from build123d import *

# Parameters (mm, degrees)
BOSS_EXTRUDE1_DEPTH = 40
SKETCH2_R           = 1.7
CUT_EXTRUDE1_DEPTH  = 28.75
SKETCH4_R           = 1.7
SKETCH4_R_2         = 11
CUT_EXTRUDE2_DEPTH  = 20
CHAMFER1_SIZE       = 1
CUT_EXTRUDE3_REACH  = 159.067
SKETCH5_R           = 3.3


with BuildPart() as part:
    # Sketch1 → Boss-Extrude1 (new body)
    with BuildSketch(Plane(origin=(0, 0, 0), x_dir=(1, 0, 0), z_dir=(0, 1, 0))):
        with BuildLine():
            Line((23.75, 120.769174208), (23.75, 134.895099729))
            Line((23.75, 134.895099729), (21.25, 134.895099729))
            Line((21.25, 134.895099729), (21.25, 123.995190528))
            ThreePointArc((21.25, 123.995190528), (17.839743095, 119.73175291), (18.223690728, 114.285714286))
            ThreePointArc((18.223690728, 114.285714286), (18.048629784, 111.396432549), (15.513167019, 110))
            Line((15.513167019, 110), (-15.513167019, 110))
            ThreePointArc((-15.513167019, 110), (-18.048629784, 111.396432549), (-18.223690728, 114.285714286))
            ThreePointArc((-18.223690728, 114.285714286), (-17.839743095, 119.73175291), (-21.25, 123.995190528))
            Line((-21.25, 123.995190528), (-21.25, 134.895099729))
            Line((-21.25, 134.895099729), (-23.75, 134.895099729))
            Line((-23.75, 134.895099729), (-23.75, 120.769174208))
            ThreePointArc((-23.75, 120.769174208), (-25, 114), (-26.25, 120.769174208))
            Line((-26.25, 120.769174208), (-26.25, 134.895099729))
            Line((-26.25, 134.895099729), (-28.75, 134.895099729))
            Line((-28.75, 134.895099729), (-28.75, 123.995190528))
            ThreePointArc((-28.75, 123.995190528), (-31.495190528, 121.25), (-32.5, 117.5))
            Line((-32.5, 117.5), (-37.5, 117.5))
            Line((-37.5, 117.5), (-42.5, 108.839745962))
            Line((-42.5, 108.839745962), (-37.000738686, 105.664745962))
            Line((-37.000738686, 105.664745962), (-47.000738686, 88.344237886))
            Line((-47.000738686, 88.344237886), (-42.670611667, 85.844237886))
            Line((-42.670611667, 85.844237886), (-31.611027254, 105))
            Line((-31.611027254, 105), (31.611027254, 105))
            Line((31.611027254, 105), (42.670611667, 85.844237886))
            Line((42.670611667, 85.844237886), (47.000738686, 88.344237886))
            Line((47.000738686, 88.344237886), (37.000738686, 105.664745962))
            Line((37.000738686, 105.664745962), (42.5, 108.839745962))
            Line((42.5, 108.839745962), (37.5, 117.5))
            Line((37.5, 117.5), (32.5, 117.5))
            ThreePointArc((32.5, 117.5), (31.495190528, 121.25), (28.75, 123.995190528))
            Line((28.75, 123.995190528), (28.75, 134.895099729))
            Line((28.75, 134.895099729), (26.25, 134.895099729))
            Line((26.25, 134.895099729), (26.25, 120.769174208))
            ThreePointArc((26.25, 120.769174208), (25, 114), (23.75, 120.769174208))
        make_face()
    extrude(amount=BOSS_EXTRUDE1_DEPTH)

    # Sketch2 → Cut-Extrude1 (cut, symmetric)
    with BuildSketch(Plane(origin=(0, 0, 0), x_dir=(0, 0, -1), z_dir=(1, 0, 0))):
        with Locations((129.445145129, 27.5)):
            Circle(SKETCH2_R)
        with Locations(Location((129.445145129, 12.5, 0), (0, 0, 180))):
            Circle(SKETCH2_R)
    extrude(amount=CUT_EXTRUDE1_DEPTH, both=True, mode=Mode.SUBTRACT)

    # Sketch4 → Cut-Extrude2 (cut)
    with BuildSketch(Plane.XY.offset(-105)):
        with Locations((-13, 33)):
            Circle(SKETCH4_R)
        with Locations((0, 20)):
            Circle(SKETCH4_R_2)
        with Locations((13, 33)):
            Circle(SKETCH4_R)
        with Locations((13, 7)):
            Circle(SKETCH4_R)
        with Locations((-13, 7)):
            Circle(SKETCH4_R)
    extrude(amount=-CUT_EXTRUDE2_DEPTH, mode=Mode.SUBTRACT)

    # Chamfer1
    chamfer1_edges = [part.edges().sort_by_distance(p)[0] for p in [
        (25, 40, -114),
        (-25, 40, -114),
    ]]
    chamfer(chamfer1_edges, length=CHAMFER1_SIZE)

    # Sketch5 → Cut-Extrude3 (cut, up to next)
    with BuildSketch(Plane(origin=(-73.504731158, 0, -42.437976321), x_dir=(-0.49999999999998673, 0, 0.8660254037844464), z_dir=(-0.8660254037844464, 0, -0.49999999999998673)), mode=Mode.PRIVATE) as cut_extrude3_sk1:
        with Locations((-63.007984945, 32.5)):
            Circle(SKETCH5_R)
    cut_extrude3_tool1 = extrude(cut_extrude3_sk1.sketch, amount=-CUT_EXTRUDE3_REACH, mode=Mode.PRIVATE) & part.part
    # Sketch5 → Cut-Extrude3 (cut, up to next)
    with BuildSketch(Plane(origin=(-73.504731158, 0, -42.437976321), x_dir=(-0.49999999999998673, 0, 0.8660254037844464), z_dir=(-0.8660254037844464, 0, -0.49999999999998673)), mode=Mode.PRIVATE) as cut_extrude3_sk2:
        with Locations((-63.007984945, 7.5)):
            Circle(SKETCH5_R)
    cut_extrude3_tool2 = extrude(cut_extrude3_sk2.sketch, amount=-CUT_EXTRUDE3_REACH, mode=Mode.PRIVATE) & part.part
    cut_extrude3_1 = cut_extrude3_tool1.solids().sort_by_distance((-42.000739, 32.5, -97.004492))[0]
    add(cut_extrude3_1, mode=Mode.SUBTRACT)
    cut_extrude3_2 = cut_extrude3_tool2.solids().sort_by_distance((-42.000739, 7.5, -97.004492))[0]
    add(cut_extrude3_2, mode=Mode.SUBTRACT)
    cut_extrude3 = cut_extrude3_1 + cut_extrude3_2  # Cut-Extrude3 as one shape, for the pattern or mirror that repeats it

    # Mirror1: Cut-Extrude3 across plane
    add(cut_extrude3.mirror(Plane(origin=(0, 0, 0), x_dir=(0, 0, 1), z_dir=(1, 0, 0))), mode=Mode.SUBTRACT)


solid = part.part
Model file for the job. Use its own axes, mm. A direction names the side the tool comes from. Round coordinates to 2 decimals unless told otherwise and drop trailing zeros. Loops run counter-clockwise (first coordinate to the right, second up) from the corner with the lowest first, then second, coordinate; pieces in that order, holes last. Notation, with made-up numbers: M 61.5,-24 L 118.5,-24 A17 ccw 118.5,-7 Z; hole C 69.5,69 d7. An arc over 180 degrees is marked long. One line per question, with ' | ' between items.
1) 3-axis set-ups, long thin cutter, end or side, ignore diameter. For faces 1 (the flat face through (-27, 20, -134.895)), 2 (the flat face through (-41.93, 19.72, -97.13)), 3 (the flat face through (-21.25, 20, -129)): which of +Z, -Z, +X, -X, +Y, -Y reach the whole face in a straight line?
Solved:
face 1: -Z, +X, -X, +Y, -Y | face 2: -X, +Y, -Y | face 3: -Z, +Y, -Y
2) Band-saw the part on C-C (x = 0). Give the cut face in (y, z).
Solved:
outline: M 0,-110 L 9,-110 L 9,-105 L 0,-105 Z; M 31,-110 L 40,-110 L 40,-105 L 31,-105 Z
3) Drill centre lines: line 1 along X through (y, z) = (2.5, -123.5); line 2 along Y through (x, z) = (13, -106.55); line 3 along X through (y, z) = (30, -115). Where is each one in solid material? Low to high.
Solved:
line 1: x = -29.5 to -26.25, -23.75 to -20.5, 20.5 to 23.75, 26.25 to 29.5 | line 2: y = 0 to 5.3, 8.7 to 31.3, 34.7 to 40 | line 3: x = -38.94 to -27.45, -22.55 to -17.93, 17.93 to 22.55, 27.45 to 38.94
4) Mould opens along X. For faces 4 (the cylindrical face through (27.482, 28.933, -130.359)), 5 (the flat face through (-28.75, 20, -130)), 6 (the cylindrical face through (18.07, 19.72, -111.43)) say: +X half, -X half, draft (parallel to the pull), parting line (faces both ways), or undercut.
Solved:
face 4: draft | face 5: -X half | face 6: undercut
5) Band-saw the part on B-B (x = -13). Give the cut face in (y, z).
Solved:
outline: M 0,-110 L 5.3,-110 L 5.3,-105 L 0,-105 Z; M 8.7,-110 L 31.3,-110 L 31.3,-105 L 8.7,-105 Z; M 34.7,-110 L 40,-110 L 40,-105 L 34.7,-105 Z
6) Band-saw the part on D-D (z = -104). Give the cut face in (x, y).
Solved:
outline: M -37.96,0 L -32.19,0 L -32.19,40 L -37.96,40 Z; M 32.19,0 L 37.96,0 L 37.96,40 L 32.19,40 Z
7) Flat gauge pins, fed straight in: pin 1 (8 mm diameter, centred on y = 19.5, z = -113.5, fed in from +X); pin 2 (15.5 mm diameter, centred on y = 12.5, z = -128, fed in from +X); pin 3 (15.5 mm diameter, centred on y = 17, z = -125, fed in from -X). Where does each tip first touch, or does it go through?
Solved:
pin 1: stops at x = 42.12 | pin 2: stops at x = 31.98 | pin 3: stops at x = -37.64
8) Band-saw the part on A-A (z = -126). Give the cut face in (x, y).
Solved:
outline: M -28.75,0 L -26.25,0 L -26.25,40 L -28.75,40 Z; M -23.75,0 L -21.25,0 L -21.25,40 L -23.75,40 Z; M 21.25,0 L 23.75,0 L 23.75,40 L 21.25,40 Z; M 26.25,0 L 28.75,0 L 28.75,40 L 26.25,40 Z
